Could you check a few things on this model? Use its own coordinates, in mm. A direction names the side the tool comes from. Round coordinates to 2 decimals unless told otherwise and drop trailing zeros. Loops run counter-clockwise (first coordinate to the right, second up) from the corner with the lowest first, then second, coordinate; pieces in that order, holes last.
Autodesk Inventor part; units mm, degrees
ref_plane "YZ Plane" through (0, 0, 0) normal (1, 0, 0) x (0, 1, 0)
ref_plane "XZ Plane" through (0, 0, 0) normal (0, 1, 0) x (-1, 0, 0)
ref_plane "XY Plane" through (0, 0, 0) normal (0, 0, 1) x (1, 0, 0)
sketch "Sketch1" plane through (0, 0, 0) normal (0, 1, 0) x (-1, 0, 0)
  line L0 (0, 0) -> (-127, 0)
  line L1 (-127, 0) -> (-127, -124.46)
  line L2 (-127, -124.46) -> (0, -124.46)
  line L3 (0, -124.46) -> (0, 0)
  dimension "d0" = 127
  dimension "d1" = 124.46
extrude "Extrusion1" add sketch "Sketch1" along normal blind 7.9375
sketch "Sketch2" plane through (0, 7.9375, 0) normal (0, 1, 0) x (1, 0, 0)
  line L0 (127, 124.46) -> (0, 124.46)
  line L1 (0, 124.46) -> (7.9248, 124.46)
  line L2 (7.9248, 124.46) -> (7.9248, 116.5352)
  line L3 (0, 0) -> (127, 0)
  line L4 (127, 0) -> (119.0752, 0)
  line L5 (119.0752, 0) -> (119.0752, 7.9248)
  line L6 (0, 0) -> (7.9248, 0)
  line L7 (7.9248, 0) -> (7.9248, 7.9248)
  line L8 (127, 124.46) -> (119.0752, 124.46)
  line L9 (119.0752, 124.46) -> (119.0752, 116.5352)
  circle A0 centre (7.9248, 116.5352) radius 3.2512
  circle A1 centre (119.0752, 7.9248) radius 3.2512
  circle A2 centre (119.0752, 116.5352) radius 3.2512
  circle A3 centre (7.9248, 7.9248) radius 3.2512
  line L10 (0, 124.46) -> (25.4, 124.46)
  line L11 (25.4, 124.46) -> (25.4, 97.3582)
  line L12 (127, 0) -> (101.6, 0)
  line L13 (0, 0) -> (25.4, 0)
  line L14 (127, 124.46) -> (101.6, 124.46)
  line L15 (101.6, 124.46) -> (101.6, 97.3582)
  circle A4 centre (25.4, 97.3582) radius 6.35
  circle A5 centre (25.4, 46.5582) radius 6.35
  circle A6 centre (101.6, 46.5582) radius 6.35
  circle A7 centre (101.6, 97.3582) radius 6.35
  line L16 (25.4, 97.3582) -> (25.4, 71.9582)
  circle A8 centre (25.4, 71.9582) radius 6.35
  circle A9 centre (101.6, 71.9582) radius 6.35
  line L17 (0, 0) -> (63.5, 0)
  circle A10 centre (63.5, 46.0502) radius 14.2875
  line L18 (63.5, 46.0502) -> (63.5, 86.741)
  circle A11 centre (63.5, 86.741) radius 11.1125
  line L19 (127, 0) -> (127, 124.46)
  dimension "d4" = 7.9248
  dimension "d5" = 7.9248
  dimension "d6" = 7.9248
  dimension "d7" = 7.9248
  dimension "d8" = 6.5024
  dimension "d9" = 6.5024
  dimension "d10" = 25.4
  dimension "d11" = 27.1018
  dimension "d12" = 25.4
  dimension "d14" = 12.7
  dimension "d15" = 25.4
  dimension "d17" = 28.575
  dimension "d18" = 40.6908
  dimension "d66" = 27.1018
  dimension "d75" = 25.4
  dimension "d76" = 37.719
  dimension "d77" = 38.1
  dimension "d78" = 38.1
  dimension "d80" = 25.4
  dimension "d81" = 25.4
  dimension "d84" = 25.4
extrude "Extrusion2" cut sketch "Sketch2" against normal blind 7.9375
fillet "Fillet1" radius 3.175 4 edges at (127, 3.9688, 0) (127, 3.9688, -124.46) (0, 3.9688, 0) (0, 3.9688, -124.46)
sketch "Sketch6" plane through (0, 7.9375, 0) normal (0, 1, 0) x (1, 0, 0)
  circle A0 centre (7.9248, 7.9248) radius 3.2512
  line L0 (7.9248, 7.9248) -> (7.9248, 28.2448)
  line L1 (7.9248, 28.2448) -> (-3.1578, 28.2448)
  line L2 (-3.1578, 28.2448) -> (0, 28.575)
  line L3 (0, 121.285) -> (0, 3.175)
  line L4 (0, 28.575) -> (0, 66.675)
  line L5 (0, 66.675) -> (-17.4752, 66.675)
  line L6 (-17.4752, 66.675) -> (-17.4752, 28.575)
  line L7 (-17.4752, 28.575) -> (0, 28.575)
  line L8 (127, 3.175) -> (127, 121.285)
  line L9 (127, 28.575) -> (144.4752, 28.575)
  line L10 (144.4752, 28.575) -> (144.4752, 66.675)
  line L11 (144.4752, 66.675) -> (127, 66.675)
  line L12 (127, 66.675) -> (127, 28.575)
  line L13 (127, 28.575) -> (127, 31.75)
  circle A1 centre (119.0752, 7.9248) radius 3.2512
  circle A2 centre (119.0752, 7.9248) radius 3.2512
  line L14 (3.175, 0) -> (123.825, 0)
  point P0 (0, 0)
  point P1 (0, 3.175)
  dimension "d47" = 3.175
  dimension "d48" = 38.1
  dimension "d49" = 17.4752
  dimension "d50" = 17.4752
  dimension "d67" = 3.175
  dimension "d69" = 38.1
  dimension "d82" = 28.575
  dimension "d83" = 28.575
extrude "Extrusion6" add sketch "Sketch6" against normal blind 7.9375 contours L7 L6 L5 L3 | L8 L11 L10 L9
sketch "Sketch7" plane through (0, 7.9375, 0) normal (0, 1, 0) x (1, 0, 0)
  line L0 (-17.4752, 28.575) -> (-17.4752, 66.675)
  line L1 (-17.4752, 66.675) -> (-8.7376, 66.675)
  line L2 (-17.4752, 66.675) -> (0, 66.675)
  line L3 (-8.7376, 66.675) -> (-8.7376, 28.575)
  line L4 (-17.4752, 28.575) -> (0, 28.575)
  line L5 (-8.7376, 66.675) -> (-8.7376, 57.15)
  line L6 (-8.7376, 57.15) -> (-8.7376, 47.625)
  line L7 (-8.7376, 47.625) -> (-8.7376, 38.1)
  circle A0 centre (-8.7376, 47.625) radius 2.54
  circle A1 centre (-8.7376, 57.15) radius 2.54
  circle A2 centre (-8.7376, 38.1) radius 2.54
  line L8 (144.4752, 66.675) -> (144.4752, 28.575)
  line L9 (144.4752, 57.15) -> (135.7376, 57.15)
  line L10 (144.4752, 47.625) -> (135.7376, 47.625)
  line L11 (144.4752, 38.1) -> (135.7376, 38.1)
  circle A3 centre (135.7376, 38.1) radius 2.54
  circle A4 centre (135.7376, 47.625) radius 2.54
  circle A5 centre (135.7376, 57.15) radius 2.54
  line L12 (144.4752, 66.675) -> (127, 66.675)
  point P0 (0, 0)
  dimension "d53" = 9.525
  dimension "d54" = 9.525
  dimension "d55" = 5.08
  dimension "d56" = 8.7376
  dimension "d70" = 9.525
  dimension "d71" = 9.525
  dimension "d72" = 9.525
extrude "Extrusion7" cut sketch "Sketch7" against normal blind 7.9375 contours A2 L3 | L3 A2 | A1 L3 | L3 A1 | A0 L3 | L3 A0 | A3 | A4 | A5
fillet "Fillet3" radius 3.175 8 edges at (127, 3.9688, -28.575) (144.4752, 3.9688, -28.575) (144.4752, 3.9688, -66.675) (-17.4752, 3.9688, -28.575) (127, 3.9688, -66.675) (0, 3.9688, -28.575) (-17.4752, 3.9688, -66.675) (0, 3.9688, -66.675)
sketch "Sketch8" plane through (0, 7.9375, 0) normal (0, 1, 0) x (1, 0, 0)
  line L0 (123.825, 124.46) -> (3.175, 124.46)
  line L1 (63.5, 124.46) -> (63.5, 105.41)
  line L2 (63.5, 105.41) -> (25.4, 105.41)
  line L3 (25.4, 105.41) -> (101.6, 105.41)
  line L4 (25.4, 105.41) -> (25.4, 124.46)
  line L5 (101.6, 105.41) -> (101.6, 124.46)
  arc A0 (25.4, 124.46) -> (101.6, 124.46) centre (63.5, 153.035) ccw
  line L6 (3.175, 0) -> (123.825, 0)
  line L7 (25.4, 0) -> (101.6, 0)
  line L8 (63.5, 0) -> (63.5, 19.05)
  arc A1 (101.6, 0) -> (25.4, 0) centre (63.5, -28.575) ccw
  point P0 (0, 0)
  dimension "d60" = 19.05
  dimension "d61" = 38.1
  dimension "d62" = 76.2
  dimension "d63" = 19.05
extrude "Extrusion8" cut sketch "Sketch8" against normal blind 7.9375 contours A0 L1 L0 | L1 A0 L0 | A1 L8 L6 | L8 A1 L6
fillet "Fillet4" radius 3.175 4 edges at (25.4, 3.9688, -124.46) (101.6, 3.9688, -124.46) (101.6, 3.9688, 0) (25.4, 3.9688, 0)
sketch "Sketch12" plane through (0, 7.9375, 0) normal (0, 1, 0) x (1, 0, 0)
  circle A0 centre (63.5, 46.0502) radius 14.2875
  circle A1 centre (63.5, 46.0502) radius 16.51
  circle A2 centre (63.5, 46.0502) radius 14.2875
  circle A3 centre (63.5, 86.741) radius 11.1125
  circle A4 centre (63.5, 86.741) radius 11.1125
  circle A5 centre (63.5, 86.741) radius 12.7
  point P0 (0, 0)
  dimension "d97" = 33.02
  dimension "d98" = 25.4
extrude "Extrusion9" cut sketch "Sketch12" against normal blind 1.5875
properties part number "2nd Plate" material "Aluminum 6061"
Item 1: Will these pins go through, and if not, where does the flat tip stop? pin 1 (2.5 mm diameter, centred on x = 134.5, y = 3, fed in from +Z) (3 decimals); pin 2 (2.5 mm diameter, centred on y = 5.5, z = -14, fed in from +X).
Results list:
pin 1: stops at z = -28.575
pin 2: stops at x = 127
Item 2: If I drill on line 1 along Z through (x, y) = (63.5, 3.25); line 2 along Z through (x, y) = (63.5, 7.45); line 3 along X through (y, z) = (4.25, -42), over which ranges is the centre line in solid material (lowest first)?
Results list:
line 1: z = -105.41 to -97.85, -75.63 to -60.34, -31.76 to -19.05
line 2: z = -105.41 to -99.44, -74.04 to -62.56, -29.54 to -19.05
line 3: x = -17.48 to 20.98, 29.82 to 49.8, 77.2 to 97.18, 106.02 to 144.48
Item 3: If we section it at C-C, the plane x = 97: Please give me the cut outline in (y, z).
Results list:
outline: (0, -119.18) - (7.94, -119.18) - (7.94, -101.74) - (0, -101.74) - close; (0, -92.98) - (7.94, -92.98) - (7.94, -76.34) - (0, -76.34) - close; (0, -67.58) - (7.94, -67.58) - (7.94, -50.94) - (0, -50.94) - close; (0, -42.18) - (7.94, -42.18) - (7.94, -5.28) - (0, -5.28) - close
Item 4: If we section it at A-A, the plane x = 63.5: Please give me the cut outline in (y, z).
Results list:
outline: (0, -105.41) - (7.94, -105.41) - (7.94, -99.44) - (6.35, -99.44) - (6.35, -97.85) - (0, -97.85) - close; (0, -75.63) - (6.35, -75.63) - (6.35, -74.04) - (7.94, -74.04) - (7.94, -62.56) - (6.35, -62.56) - (6.35, -60.34) - (0, -60.34) - close; (0, -31.76) - (6.35, -31.76) - (6.35, -29.54) - (7.94, -29.54) - (7.94, -19.05) - (0, -19.05) - close
Item 5: If we section it at B-B, the plane z = -57.15: Please give me the cut outline in (x, y).
Results list:
outline: (-17.48, 0) - (-11.28, 0) - (-11.28, 7.94) - (-17.48, 7.94) - close; (-6.2, 0) - (54.5, 0) - (54.5, 6.35) - (51.28, 6.35) - (51.28, 7.94) - (-6.2, 7.94) - close; (72.5, 0) - (133.2, 0) - (133.2, 7.94) - (75.72, 7.94) - (75.72, 6.35) - (72.5, 6.35) - close; (138.28, 0) - (144.48, 0) - (144.48, 7.94) - (138.28, 7.94) - close
Item 6: We'd pull the mould along X, two halves only. Please class faces 4 (the flat face through (13, 4, 0)), 5 (the cylindrical face through (127.905, 3.913, -27.62)), 6 (the cylindrical face through (-10.61, 4.024, -39.817)), 7 (the cylindrical face through (-16.57, 3.91, -65.72)): released by +X, released by -X, zero draft, split by the parting line, or undercut.
Results list:
face 4: zero draft
face 5: released by +X
face 6: undercut
face 7: released by -X
Item 7: For faces 1 (the flat face through (127, 4, -14)), 2 (the cylindrical face through (64.097, 4.024, -19.046)), 3 (the flat face through (59, 6.35, -60)), which set-ups out of +Z, -Z, +X, -X, +Y, -Y let a thin tool reach every point of the face, with its end or its side?
Results list:
face 1: +Z, +X, +Y, -Y
face 2: +Z, +Y, -Y
face 3: +Y
Item 8: If we section it at D-D, the plane z = -38.1: Please give me the cut outline in (x, y), then the cut area to 3 significant figures.
Results list:
outline: (-17.48, 0) - (-11.28, 0) - (-11.28, 7.94) - (-17.48, 7.94) - close; (-6.2, 0) - (51.63, 0) - (51.63, 6.35) - (49.03, 6.35) - (49.03, 7.94) - (-6.2, 7.94) - close; (75.37, 0) - (133.2, 0) - (133.2, 7.94) - (77.97, 7.94) - (77.97, 6.35) - (75.37, 6.35) - close; (138.28, 0) - (144.48, 0) - (144.48, 7.94) - (138.28, 7.94) - close
area: 1,010 mm2
